Solid Edge part; units mm, degrees
sketch "Sketch1" plane through (0, 0, 0) normal (0, 0, 1) x (1, 0, 0)
  line L0 (-200, -90) -> (200, -90)
  line L1 (200, -90) -> (200, 90)
  line L2 (200, 90) -> (-200, 90)
  line L3 (-200, 90) -> (-200, -90)
  line L4 (-150, -81) -> (-170, -81)
  line L5 (-170, -81) -> (-170, -85)
  line L6 (-170, -85) -> (-150, -85)
  line L7 (-150, -85) -> (-150, -81)
  line L8 (-90, -85) -> (-70, -85)
  line L9 (-70, -85) -> (-70, -81)
  line L10 (-70, -81) -> (-90, -81)
  line L11 (-90, -81) -> (-90, -85)
  line L12 (-10, -85) -> (10, -85)
  line L13 (10, -85) -> (10, -81)
  line L14 (10, -81) -> (-10, -81)
  line L15 (-10, -81) -> (-10, -85)
  line L16 (70, -85) -> (90, -85)
  line L17 (90, -85) -> (90, -81)
  line L18 (90, -81) -> (70, -81)
  line L19 (70, -81) -> (70, -85)
  line L20 (150, -85) -> (170, -85)
  line L21 (170, -85) -> (170, -81)
  line L22 (170, -81) -> (150, -81)
  line L23 (150, -81) -> (150, -85)
  line L24 (160, 100) -> (120, 100)
  line L25 (120, 100) -> (120, 90)
  line L26 (120, 90) -> (160, 90)
  line L27 (160, 90) -> (160, 100)
  line L28 (80, 100) -> (40, 100)
  line L29 (40, 100) -> (40, 90)
  line L30 (40, 90) -> (80, 90)
  line L31 (80, 90) -> (80, 100)
  line L32 (0, 100) -> (-40, 100)
  line L33 (-40, 100) -> (-40, 90)
  line L34 (-40, 90) -> (0, 90)
  line L35 (0, 90) -> (0, 100)
  line L36 (-80, 100) -> (-120, 100)
  line L37 (-120, 100) -> (-120, 90)
  line L38 (-120, 90) -> (-80, 90)
  line L39 (-80, 90) -> (-80, 100)
  line L40 (-160, 100) -> (-200, 100)
  line L41 (-200, 100) -> (-200, 90)
  line L42 (-200, 90) -> (-160, 90)
  line L43 (-160, 90) -> (-160, 100)
  line L44 (-191, 25) -> (-191, 45)
  line L45 (-191, 45) -> (-195, 45)
  line L46 (-195, 45) -> (-195, 25)
  line L47 (-195, 25) -> (-191, 25)
  line L48 (-195, -35) -> (-195, -55)
  line L49 (-195, -55) -> (-191, -55)
  line L50 (-191, -55) -> (-191, -35)
  line L51 (-191, -35) -> (-195, -35)
  line L52 (191, -35) -> (191, -55)
  line L53 (191, -55) -> (195, -55)
  line L54 (195, -55) -> (195, -35)
  line L55 (195, -35) -> (191, -35)
  line L56 (195, 25) -> (195, 45)
  line L57 (195, 45) -> (191, 45)
  line L58 (191, 45) -> (191, 25)
  line L59 (191, 25) -> (195, 25)
extrude "Protrusion1" add sketch "Sketch1" along normal blind 4
The listing builds one solid part. Answer for the finished solid, in the listing's coordinates (mm). Give positions to 0.01 mm unless a question says otherwise; leave off trailing zeros. Order: outer loops, then holes, each group sorted by start corner. A loop starts at its lowest first (then second) coordinate and runs counter-clockwise, first axis right, second up. Notation, with made-up numbers: M 4.5,37 L 34.5,37 A20 ccw 34.5,73 Z; hole C 6,77 d6. An arc over 180 degrees is marked long. Put each result on its own line as item: value. Start each with the question number.
Item 1: Find the intervals of material crossed by line 1 along X through (y, z) = (-51.5, 0.3); line 2 along Y through (x, z) = (75.5, 2.1); line 3 along Y through (x, z) = (167.5, 1.75), in increasing order.
Item 2: The part is cut by section B-B, the plane z = 2.9. State how many separate pieces and enclosed holes the cut face has, and give its area (3 significant figures).
Item 3: The part is cut by section A-A, the plane y = -47. Determine the outline of the cut face in (x, z).
Item 4: A flat-ended cylindrical pin translates along its axis: P1, Ø2, axis at x = 102.5, z = 2, coming from the +Y side. Find the tip coordinate at first contact, or state that the pin passes through.
Item 5: The part is cut by section C-C, the plane x = 27.5. Determine the outline of the cut face in (y, z), and give its area (3 significant figures).
Answer key:
1. line 1: x = -200 to -195, -191 to 191, 195 to 200
1. line 2: y = -90 to -85, -81 to 100
1. line 3: y = -90 to -85, -81 to 90
2. separate pieces: 1
2. enclosed holes: 9
2. area: 73,300 mm²
3. outline: M -200,0 L -195,0 L -195,4 L -200,4 Z; M -191,0 L 191,0 L 191,4 L -191,4 Z; M 195,0 L 200,0 L 200,4 L 195,4 Z
4. P1: stops at y = 90
5. outline: M -90,0 L 90,0 L 90,4 L -90,4 Z
5. area: 720 mm²
